Verification items for the finished model (mm, model axes). Face numbers are marked on the shaded views. A direction names the side the tool comes from. Give positions to 0.01 mm unless a question says otherwise; leave off trailing zeros. Loops run counter-clockwise (first coordinate to the right, second up) from the corner with the lowest first, then second, coordinate; pieces in that order, holes last. Notation, with made-up numbers: M 89.25,86.25 L 126.25,86.25 A26 cw 126.25,117.25 Z; hole C 87,-36 d8. An arc over 180 degrees is marked long. Put each result on its own line as item: value. Start each with the question number.
from build123d import *

# Parameters (mm, degrees)
SKETCH1_W               = 63.5
SKETCH1_H               = 50.8
BOSS_EXTRUDE1_DEPTH     = 20.32
SKETCH2_R               = 7.493
CUT_EXTRUDE1_DEPTH      = 11.9888
SKETCH3_W               = 31.75
SKETCH3_H               = 1.778
CUT_EXTRUDE2_DEPTH      = 11.9888
SKETCH9_R               = 1.9939
CUT_EXTRUDE3_DEPTH      = 11.9888
CUT_EXTRUDE4_START      = -6.331204
SKETCH10_R              = 7.493
CUT_EXTRUDE4_DEPTH      = 6.331204
SKETCH11_R              = 2.5527
CUT_EXTRUDE5_DEPTH      = 21.32
MIRROR2_COPY_1_SKETCH_R = 2.5527
MIRROR2_COPY_1_DEPTH    = 21.32


with BuildPart() as part:
    # Sketch1 → Boss-Extrude1 (new body)
    with BuildSketch(Plane.XY):
        Rectangle(SKETCH1_W, SKETCH1_H)
    extrude(amount=BOSS_EXTRUDE1_DEPTH)

    # Sketch2 → Cut-Extrude1 (cut)
    with BuildSketch(Plane.XY.offset(20.32)):
        Circle(SKETCH2_R)
    extrude(amount=-CUT_EXTRUDE1_DEPTH, mode=Mode.SUBTRACT)

    # Sketch3 → Cut-Extrude2 (cut)
    with BuildSketch(Plane.XY.offset(20.32)):
        with Locations((15.875, 0)):
            Rectangle(SKETCH3_W, SKETCH3_H)
    extrude(amount=-CUT_EXTRUDE2_DEPTH, mode=Mode.SUBTRACT)

    # Sketch9 → Cut-Extrude3 (cut)
    with BuildSketch(Plane.XY.offset(8.3312)):
        Circle(SKETCH9_R)
    extrude(amount=-CUT_EXTRUDE3_DEPTH, mode=Mode.SUBTRACT)

    # Sketch10 → Cut-Extrude4 (cut)
    with BuildSketch(Plane(origin=(0, 0, 0), x_dir=(-1, 0, 0), z_dir=(0, 0, -1)).offset(CUT_EXTRUDE4_START)):
        Circle(SKETCH10_R)
    extrude(amount=CUT_EXTRUDE4_DEPTH, mode=Mode.SUBTRACT)

    # Sketch11 → Cut-Extrude5 (cut, through all)
    with BuildSketch(Plane.XY.offset(20.32)):
        with Locations((-25.4, 19.05)):
            Circle(SKETCH11_R)
    cut_extrude5 = extrude(amount=-CUT_EXTRUDE5_DEPTH, mode=Mode.SUBTRACT)

    # Mirror1: Cut-Extrude5 across plane
    add(cut_extrude5.mirror(Plane(origin=(0, 0, 0), x_dir=(0, 0, 1), z_dir=(1, 0, 0))), mode=Mode.SUBTRACT)

    # Mirror2: Cut-Extrude5 across plane
    add(cut_extrude5.mirror(Plane.ZX), mode=Mode.SUBTRACT)

    # Mirror2 copy 1 sketch → Mirror2 copy 1 (cut, through all)
    with BuildSketch(Plane(origin=(0, 0, 20.32), x_dir=(-1, 0, 0), z_dir=(0, 0, 1))):
        with Locations((-25.4, 19.05)):
            Circle(MIRROR2_COPY_1_SKETCH_R)
    extrude(amount=-MIRROR2_COPY_1_DEPTH, mode=Mode.SUBTRACT)


solid = part.part
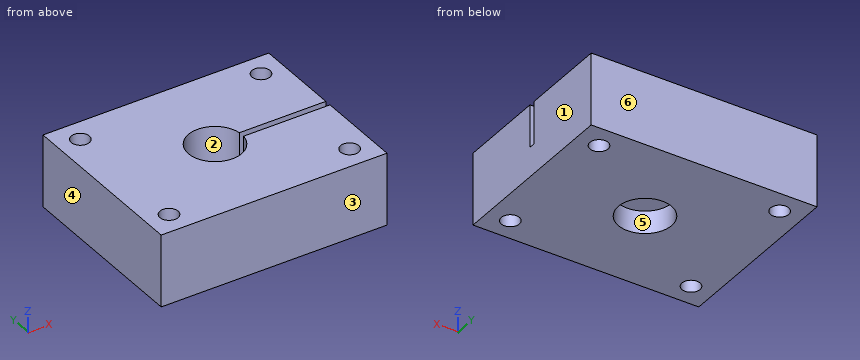
Q1. Release check for a two-part mould opening along X. For the marked faces 1, 2, 3 and 4 record: pulls with the +X half, pulls with the -X half, needs draft (parallel to the pull), parting line crosses it, or undercut.
Q2. Scan lines: L1, parallel to Y at x = 25.4, z = 16.25; L2, parallel to Y at x = -25.4, z = 5.75; L3, parallel to Y at x = 12, z = 19.25. Record each from-to range of solid material in increasing order.
Q3. Go/stop test with flat-tipped pins: pin 1 (4.5 mm diameter, centred on x = -25.4, y = 19.05, fed in from +Z); pin 2 (4 mm diameter, centred on x = -4.5, y = -14.5, fed in from -Z); pin 3 (4.5 mm diameter, centred on x = 0, y = 0, fed in from -Z); pin 4 (9 mm diameter, centred on x = 0, y = 0, fed in from +Z). Record where each tip stops, or that it passes through.
Q4. Set-up check for the marked faces 5 and 6: record each of +Z, -Z, +X, -X, +Y, -Y from which the full face is reachable in a straight line by a thin tool's end or side.
Q5. Cross-section at C-C, the plane z = 2. Record the boundary of the cut face in (x, y).
Q6. Cross-section at B-B, the plane y = -19.05. Record the boundary of the cut face in (x, z), then the cut area to 3 significant figures.
Q7. Cross-section at D-D, the plane x = -25.4. Record the boundary of the cut face in (y, z).
Q8. Cross-section at A-A, the plane x = 0. Record the boundary of the cut face in (y, z), then the cut area to 3 significant figures.
Ans:
1. face 1: pulls with the +X half
1. face 2: undercut
1. face 3: needs draft
1. face 4: pulls with the -X half
2. L1: y = -25.4 to -21.6, -16.5 to -0.89, 0.89 to 16.5, 21.6 to 25.4
2. L2: y = -25.4 to -21.6, -16.5 to 16.5, 21.6 to 25.4
2. L3: y = -25.4 to -0.89, 0.89 to 25.4
3. pin 1: passes through
3. pin 2: stops at z = 0
3. pin 3: stops at z = 6.33
3. pin 4: stops at z = 8.33
4. face 5: -Z
4. face 6: +Z, -Z, +X, -X, +Y
5. outline: M -31.75,-25.4 L 31.75,-25.4 L 31.75,25.4 L -31.75,25.4 Z; hole C -25.4,-19.05 d5.11; hole C -25.4,19.05 d5.11; hole C 0,0 d14.99; hole C 25.4,-19.05 d5.11; hole C 25.4,19.05 d5.11
6. outline: M -31.75,0 L -27.95,0 L -27.95,20.32 L -31.75,20.32 Z; M -22.85,0 L 22.85,0 L 22.85,20.32 L -22.85,20.32 Z; M 27.95,0 L 31.75,0 L 31.75,20.32 L 27.95,20.32 Z
6. area: 1,080 mm^2
7. outline: M -25.4,0 L -21.6,0 L -21.6,20.32 L -25.4,20.32 Z; M -16.5,0 L 16.5,0 L 16.5,20.32 L -16.5,20.32 Z; M 21.6,0 L 25.4,0 L 25.4,20.32 L 21.6,20.32 Z
8. outline: M -25.4,0 L -7.49,0 L -7.49,6.33 L -1.99,6.33 L -1.99,8.33 L -7.49,8.33 L -7.49,20.32 L -25.4,20.32 Z; M 1.99,6.33 L 7.49,6.33 L 7.49,0 L 25.4,0 L 25.4,20.32 L 7.49,20.32 L 7.49,8.33 L 1.99,8.33 Z
8. area: 750 mm^2
